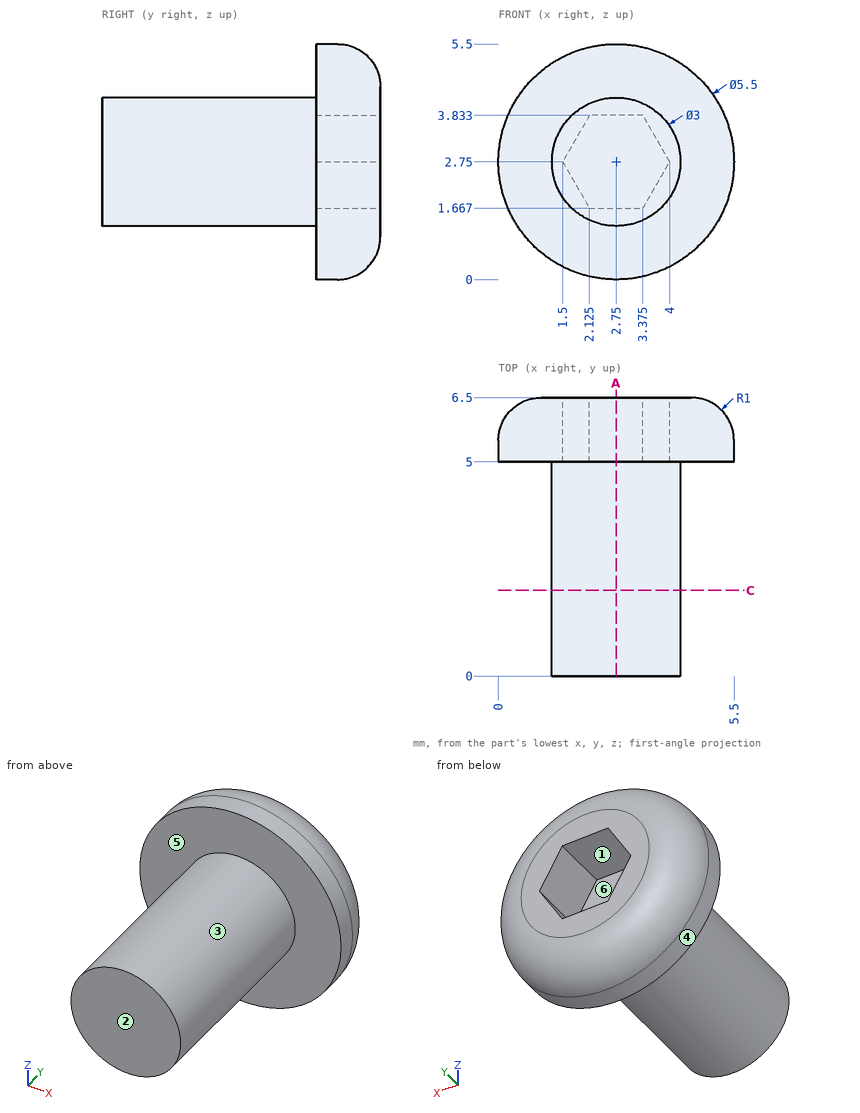
Job drawing, mm, ordinate dimensions from the low corner. One solid piece. A direction names the side the tool comes from. Round coordinates to 2 decimals unless told otherwise and drop trailing zeros. Loops run counter-clockwise (first coordinate to the right, second up) from the corner with the lowest first, then second, coordinate; pieces in that order, holes last. Notation, with made-up numbers: (-8, 74) -> (6, 74) arc R21 ccw to (6, 97) -> close; hole circle Ø1 at (63, 12.5). An arc over 180 degrees is marked (long way). Use CSV: the item, a comma, the result in double quotes. Start each with the question number.
Q1. Flat gauge pins, fed straight in: pin 1 Ø1.5 at (x, y) = (1, 5.5) entering from +Z; pin 2 Ø0.6 at (x, y) = (2.5, 6) entering from +Z. Where does each tip first touch, or does it go through?
Q2. Drill centre lines: L1, parallel to Y at x = 1.9, z = 2.45; L2, parallel to Y at x = 4.45, z = 2.8; L3, parallel to Z at x = 2.7, y = 2. Where is each one in solid material? Low to high.
Q3. Mould opens along X. For the marked faces 4, 5 and 6 say: +X half, -X half, draft (parallel to the pull), parting line (faces both ways), or undercut.
Q4. Which spindle directions (+Z, -Z, +X, -X, +Y, -Y) get a long thin tool onto all of the face, cutting with end or side? Do the marked faces 1, 2 and 3. Say none if no direction does.
Q5. Saw through at A-A on x = 2.75. Give the cut face in (y, z).
Q6. Saw through at C-C on y = 2. Give the cut face in (x, z).
Solutions:
1,pin 1,"stops at z = 5.31"
1,pin 2,"stops at z = 5.47"
2,L1,"y = 0 to 5"
2,L2,"y = 5 to 6.5"
2,L3,"z = 1.25 to 4.25"
3,face 4,"parting line"
3,face 5,"draft"
3,face 6,"undercut"
4,face 1,"+Y"
4,face 2,"+Z, -Z, +X, -X, -Y"
4,face 3,"-Y"
5,outline,"(0, 1.25) -> (5, 1.25) -> (5, 0) -> (5.5, 0) arc R1 ccw to (6.5, 1) -> (6.5, 1.67) -> (5, 1.67) -> (5, 3.83) -> (6.5, 3.83) -> (6.5, 4.5) arc R1 ccw to (5.5, 5.5) -> (5, 5.5) -> (5, 4.25) -> (0, 4.25) -> close"
6,outline,"circle Ø3 at (2.75, 2.75)"
